CAD build for the part. Positions are in the model's coordinates, mm. Coordinates: 2 decimals unless noted, no trailing zeros. Order: outer loops, then holes, each group sorted by start corner. A loop starts at its lowest first (then second) coordinate and runs counter-clockwise, first axis right, second up. Notation, with made-up numbers: (41, 38) - (48, 38) arc R8 ccw to (48, 50) - close; hole circle Ø11 at (6, -32.5). An arc over 180 degrees is marked (long way). Return JSON: item names as keys, results as strings.
from build123d import *

# Parameters (mm, degrees)
F0_W     = 787.4
F0_H     = 50.8
F1_DEPTH = 25.4
F3_DEPTH = 25.4
F5_DEPTH = 25.4


with BuildPart() as f1:
    # F0 (on Front) → F1 (new body)
    with BuildSketch(Plane.XZ):
        with Locations((-160.468298, -86.47181)):
            Rectangle(F0_W, F0_H)
    extrude(amount=F1_DEPTH)

    # F2 (on face) → F3 (cut)
    with BuildSketch(Plane.XZ.offset(25.4)):
        Polygon((182.431702, -111.87181), (233.231702, -111.87181), (233.231702, -61.07181), align=None)
    extrude(amount=-F3_DEPTH, mode=Mode.SUBTRACT)

    # F4 (on face) → F5 (cut)
    with BuildSketch(Plane.XZ.offset(25.4)):
        Polygon((-554.168298, -61.07181), (-554.168298, -111.87181), (-503.368298, -111.87181), align=None)
    extrude(amount=-F5_DEPTH, mode=Mode.SUBTRACT)


solid = f1.part
Item 1: Wall check: L1, parallel to X at y = -2, z = -76; L2, parallel to X at y = -19, z = -108.5. Give the ranges that are in metal, low to high. Write a range as [from, to].
Findings below:
{"L1": "x = [-539.24, 218.3]", "L2": "x = [-506.74, 185.8]"}
Item 2: Band-saw the part on B-B, the plane z = -76. List the corners of the cut face in (x, y), then the cut area to 3 significant figures.
Findings below:
{"outline": "(-539.24, -25.4) - (218.3, -25.4) - (218.3, 0) - (-539.24, 0) - close", "area": "19,200 mm²"}
Item 3: Drop flat-ended pins along their axis: P1, Ø3, axis at y = -12, z = -84.5, coming from the -X side; P2, Ø1, axis at y = -13.5, z = -78, coming from the +X side; P3, Ø1.5, axis at y = -13, z = -82.5, coming from the -X side. Give the stop position or say it passes through.
Findings below:
{"P1": "stops at x = -532.24", "P2": "stops at x = 216.8", "P3": "stops at x = -533.49"}
Item 4: Band-saw the part on A-A, the plane y = -12. List the corners of the cut face in (x, z), then the cut area to 3 significant figures.
Findings below:
{"outline": "(-554.17, -61.07) - (-503.37, -111.87) - (182.43, -111.87) - (233.23, -61.07) - close", "area": "37,400 mm²"}
